```python
from build123d import *

# Parameters (mm, degrees)
F0_W     = 15
F0_H     = 2.5
F1_DEPTH = 3


with BuildPart() as f1:
    # F0 (on Front) → F1 (new body)
    with BuildSketch(Plane.XZ):
        Polygon((54.065418, -36), (84.065418, -36), (84.065418, 54), (69.065418, 54), (69.065418, 57.5), (84.065418, 57.5), (84.065418, 60), (-50.934582, 60), (-50.934582, 57.5), (-50.934582, 54), (-65.934582, 54), (-65.934582, -36), (-35.934582, -36), (-35.934582, 0), (54.065418, 0), align=None)
        with Locations((-58.434582, 58.75)):
            Rectangle(F0_W, F0_H)
    extrude(amount=F1_DEPTH)


solid = f1.part
```
Check sheet for the modelled part. Datum: model origin and axes. Units: mm. A direction names the side the tool comes from. Give positions to 0.01 mm unless a question says otherwise; leave off trailing zeros. Order: outer loops, then holes, each group sorted by start corner. A loop starts at its lowest first (then second) coordinate and runs counter-clockwise, first axis right, second up. Notation, with made-up numbers: (-18.75, 55) -> (23.25, 55) arc R15 cw to (23.25, 73) -> close; hole circle Ø1 at (44, 63). An arc over 180 degrees is marked (long way). Return JSON: item names as keys, results as strings.
1. Cross-section at B-B, the plane y = -1.7. Record the cut outline in (x, z).
From the geometry:
{"outline": "(-65.93, -36) -> (-35.93, -36) -> (-35.93, 0) -> (54.07, 0) -> (54.07, -36) -> (84.07, -36) -> (84.07, 54) -> (69.07, 54) -> (69.07, 57.5) -> (84.07, 57.5) -> (84.07, 60) -> (-65.93, 60) -> (-65.93, 57.5) -> (-50.93, 57.5) -> (-50.93, 54) -> (-65.93, 54) -> close"}
2. Cross-section at A-A, the plane z = -28.5. Record the cut outline in (x, y), plus the area to 3 significant figures.
From the geometry:
{"outline": "(-65.93, -3) -> (-35.93, -3) -> (-35.93, 0) -> (-65.93, 0) -> close; (54.07, -3) -> (84.07, -3) -> (84.07, 0) -> (54.07, 0) -> close", "area": "180 mm^2"}
3. Material ranges on probe 1 along X at (y, z) = (-2.1, -30); probe 2 along Z at (x, y) = (38, -2.55), recorded low to high. Write a range as [from, to].
From the geometry:
{"probe 1": "[-65.93, -35.93], [54.07, 84.07]", "probe 2": "[0, 60]"}
4. Set-up check for faces 4 (the flat face through (-58, -1, 54)), 5 (the flat face through (10, -1, 60)), 6 (the flat face through (84.065, -1, 8)), 7 (the flat face through (77, -1, 54)), 8 (the flat face through (54.065, -1, -18)): record each of +Z, -Z, +X, -X, +Y, -Y from which the full face is reachable in a straight line by a thin tool's end or side.
From the geometry:
{"face 4": "-X, +Y, -Y", "face 5": "+Z, +X, -X, +Y, -Y", "face 6": "+Z, -Z, +X, +Y, -Y", "face 7": "+X, +Y, -Y", "face 8": "-Z, +Y, -Y"}
5. Go/stop test with flat-tipped pins: P1, Ø0.9, axis at y = -2, z = 55.5, coming from the -X side; P2, Ø1.5, axis at x = 11.5, y = -1.5, coming from the -Z side; P3, Ø6, axis at x = 56.5, z = 8, coming from the +Y side. Record where each tip stops, or that it passes through.
From the geometry:
{"P1": "x = -50.93", "P2": "z = 0", "P3": "y = 0"}
6. Mould release check, pull along X, two halves, no side actions. Record for faces 1 (the flat face through (-65.935, -1, 10)), 2 (the flat face through (-59, -1, 57.5)), 3 (the flat face through (-35.935, -1, -18)): +X half, -X half, draft (parallel to the pull), parting line (faces both ways), or undercut.
From the geometry:
{"face 1": "-X half", "face 2": "draft", "face 3": "undercut"}
7. Cross-section at C-C, the plane x = -24. Record the cut outline in (y, z), plus the area to 3 significant figures.
From the geometry:
{"outline": "(-3, 0) -> (0, 0) -> (0, 60) -> (-3, 60) -> close", "area": "180 mm^2"}
